Here's how the part is built. I have some questions about the finished solid (model axes, mm). Face numbers are marked on the shaded views. A direction names the side the tool comes from. Give positions to 0.01 mm unless a question says otherwise; leave off trailing zeros. Write each loop counter-clockwise with the first axis right and the second up, starting at its lowest first coordinate (ties: lowest second). Pieces come first, ordered by that corner, then holes. Notation, with made-up numbers: (89.25, 79.25) -> (136.25, 79.25) arc R24 ccw to (136.25, 99.25) -> close; hole circle Ø8 at (74, -18). An arc over 180 degrees is marked (long way). Put each result on its own line as item: value. Start each with the question number.
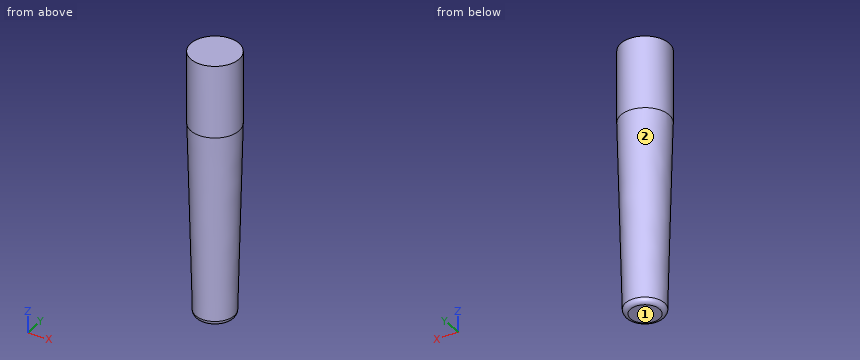
from build123d import *

# Parameters (mm, degrees)
F2_R     = 5
F0_R     = 4
F4_R     = 1
F5_R     = 5
F6_DEPTH = 15


with BuildPart() as f3:
    # F2 (on offset) → F3 section 0
    with BuildSketch(Plane.XY.offset(40)):
        Circle(F2_R)
    # F0 (on Top) → F3 section 1
    with BuildSketch(Plane.XY):
        Circle(F0_R)
    loft()

    # F4
    f4_edges = [f3.edges().sort_by_distance(p)[0] for p in [
        (-4, 0, 0),
    ]]
    fillet(f4_edges, radius=F4_R)

    # F5 (on face) → F6 (join)
    with BuildSketch(Plane.XY.offset(40)):
        Circle(F5_R)
    extrude(amount=F6_DEPTH)


solid = f3.part
1) I'm going to push flat-ended pins straight in: pin 1 Ø3 at (x, z) = (-1, 37) entering from +Y; pin 2 Ø1.5 at (x, z) = (4, 30) entering from +Y; pin 3 Ø1.5 at (y, z) = (0.5, 28.5) entering from +X. Where does each tip first touch, or does it pass through?
2) I need wall thicknesses on probe 1 along Y at (x, z) = (2.25, 24.5); probe 2 along X at (y, z) = (-3, 7.5); probe 3 along X at (y, z) = (-1, 3.5). Which ranges of each line are inside material? Lowest first, please.
3) I want a section at A-A, the plane x = 0. Write out the boundary of the cut face in (y, z) (3 decimals), and give its area (3 significant figures).
4) I want a section at C-C, the plane z = 10. Write out the boundary of the cut face in (x, y).
5) Which directions (+Z, -Z, +X, -X, +Y, -Y) give clear straight access to the entire face, cutting with the end or side of a thin tool? Please do the marked faces 1 and 2.
6) I want a section at B-B, the plane z = 48. Write out the boundary of the cut face in (x, y), and give its area (3 significant figures).
Established:
1. pin 1: stops at y = 4.95
1. pin 2: stops at y = 3.46
1. pin 3: stops at x = 4.73
2. probe 1: y = -4.03 to 4.03
2. probe 2: x = -2.92 to 2.92
2. probe 3: x = -3.96 to 3.96
3. outline: (-5, 40) -> (-4.024, 0.975) arc R1 ccw to (-3.025, 0) -> (3.025, 0) arc R1 ccw to (4.024, 0.975) -> (5, 40) -> (5, 55) -> (-5, 55) -> close
3. area: 510 mm2
4. outline: circle Ø8.5 at (0, 0)
5. face 1: -Z, +X, -X, +Y, -Y
5. face 2: -Z
6. outline: circle Ø10 at (0, 0)
6. area: 78.5 mm2
